```python
from build123d import *

# Parameters (mm, degrees)
CROQUIS1_W              = 10
CROQUIS1_H              = 8.5
SALIENTE_EXTRUIR1_DEPTH = 9.4
CROQUIS2_W              = 10
CROQUIS2_H              = 7
CORTAR_EXTRUIR1_DEPTH   = 6.2
CROQUIS3_W              = 0.25
CROQUIS3_H              = 8
CORTAR_EXTRUIR2_DEPTH   = 10
CROQUIS4_W              = 3
CROQUIS4_H              = 0.5
CORTAR_EXTRUIR3_DEPTH   = 10
CROQUIS5_W              = 4
CROQUIS5_H              = 1
CORTAR_EXTRUIR4_DEPTH   = 10
CROQUIS6_R              = 0.57
SALIENTE_EXTRUIR2_DEPTH = 7.3
REDONDEO2_R             = 0.5
CROQUIS7_W              = 1
CROQUIS7_H              = 1.5
CORTAR_EXTRUIR5_DEPTH   = 14.8
CROQUIS8_W              = 3
CROQUIS8_H              = 3.2
CORTAR_EXTRUIR6_DEPTH   = 1.5
CORTAR_EXTRUIR7_DEPTH   = 10


with BuildPart() as part:
    # Croquis1 → Saliente-Extruir1 (new body)
    with BuildSketch(Plane(origin=(0, 0, 0), x_dir=(1, 0, 0), z_dir=(0, 1, 0))):
        Rectangle(CROQUIS1_W, CROQUIS1_H)
    extrude(amount=SALIENTE_EXTRUIR1_DEPTH)

    # Croquis2 → Cortar-Extruir1 (cut)
    with BuildSketch(Plane(origin=(0, 9.4, 0), x_dir=(1, 0, 0), z_dir=(0, 1, 0))):
        with Locations((0, 0.75)):
            Rectangle(CROQUIS2_W, CROQUIS2_H)
    extrude(amount=-CORTAR_EXTRUIR1_DEPTH, mode=Mode.SUBTRACT)

    # Croquis3 → Cortar-Extruir2 (cut)
    with BuildSketch(Plane.ZY.offset(5)):
        with Locations((4.125, 4)):
            Rectangle(CROQUIS3_W, CROQUIS3_H)
    extrude(amount=-CORTAR_EXTRUIR2_DEPTH, mode=Mode.SUBTRACT)

    # Croquis4 → Cortar-Extruir3 (cut)
    with BuildSketch(Plane(origin=(0, 0, -4.25), x_dir=(-1, 0, 0), z_dir=(0, 0, -1))):
        with Locations((0, 0.25)):
            Rectangle(CROQUIS4_W, CROQUIS4_H)
    extrude(amount=-CORTAR_EXTRUIR3_DEPTH, mode=Mode.SUBTRACT)

    # Croquis5 → Cortar-Extruir4 (cut)
    with BuildSketch(Plane.ZY.offset(5)):
        with Locations((0.75, 0.5)):
            Rectangle(CROQUIS5_W, CROQUIS5_H)
    extrude(amount=-CORTAR_EXTRUIR4_DEPTH, mode=Mode.SUBTRACT)

    # Croquis6 → Saliente-Extruir2 (add, symmetric)
    with BuildSketch(Plane(origin=(0, 3.6, 0), x_dir=(1, 0, 0), z_dir=(0, 1, 0))):
        with Locations(Location((-2.5, -0.5, 0), (0, 0, 270))):
            Circle(CROQUIS6_R)
        with Locations(Location((2.5, -0.5, 0), (0, 0, 270))):
            Circle(CROQUIS6_R)
    extrude(amount=SALIENTE_EXTRUIR2_DEPTH, both=True)

    # Redondeo2
    redondeo2_edges = [part.edges().sort_by_distance(p)[0] for p in [
        (2.5, -3.7, -0.07),
        (2.5, 10.9, -0.07),
        (-2.5, -3.7, -0.07),
        (-2.5, 10.9, -0.07),
    ]]
    fillet(redondeo2_edges, radius=REDONDEO2_R)

    # Croquis7 → Cortar-Extruir5 (cut)
    with BuildSketch(Plane(origin=(0, 9.4, 0), x_dir=(1, 0, 0), z_dir=(0, 1, 0))):
        with Locations((-4.5, -3.5)):
            Rectangle(CROQUIS7_W, CROQUIS7_H)
        with Locations((4.5, -3.5)):
            Rectangle(CROQUIS7_W, CROQUIS7_H)
    extrude(amount=-CORTAR_EXTRUIR5_DEPTH, mode=Mode.SUBTRACT)

    # Croquis8 → Cortar-Extruir6 (cut)
    with BuildSketch(Plane.XY.offset(4)):
        with Locations((0, 1.6)):
            Rectangle(CROQUIS8_W, CROQUIS8_H)
    extrude(amount=-CORTAR_EXTRUIR6_DEPTH, mode=Mode.SUBTRACT)

    # Croquis9 → Cortar-Extruir7 (cut)
    with BuildSketch(Plane.ZY.offset(4)):
        Polygon((4.25, 8.6), (4.25, 9.4), (3.85, 9.4), align=None)
        Polygon((2.75, 8.5), (2.75, 9.4), (3.15, 9.4), align=None)
    extrude(amount=-CORTAR_EXTRUIR7_DEPTH, mode=Mode.SUBTRACT)


solid = part.part
```
Part model, mm, in its own coordinate system. A direction names the side the tool comes from. Round coordinates to 2 decimals unless told otherwise and drop trailing zeros. Loops run counter-clockwise (first coordinate to the right, second up) from the corner with the lowest first, then second, coordinate; pieces in that order, holes last. Notation, with made-up numbers: (49.25, 79.5) -> (95.25, 79.5) arc R20 cw to (95.25, 111.5) -> close; hole circle Ø6 at (-40, 45). An arc over 180 degrees is marked (long way). Use CSV: the item, a comma, the result in double quotes. Start each with the question number.
1) Cut at C-C, the plane x = -3.25. Write the cut outline in (y, z).
2) Drop flat-ended pins along their axis: P1, Ø1.1, axis at x = 4.5, y = 2.5, coming from the +Z side; P2, Ø1.4, axis at x = -2.5, z = 3.5, coming from the -Y side; P3, Ø3.5, axis at x = -1, z = -2, coming from the +Y side. Give the stop position or say it passes through.
3) Cut at B-B, the plane y = 6.5. Write the cut outline in (x, z).
4) Which spindle directions (+Z, -Z, +X, -X, +Y, -Y) get a long thin tool onto all of the face, cutting with end or side? Do faces 4 (the flat face through (-0.056, 8.956, 2.953)), 5 (the flat face through (3, 0, 3)), 6 (the flat face through (3, 0, -3)), 7 (the cylindrical face through (-2.85, -1.07, 0.05)). Say none if no direction does.
5) Cut at A-A, the plane x = -0.5. Write the cut outline in (y, z).
6) Wall check: L1, parallel to X at y = -0.5, z = 0.5; L2, parallel to Y at x = 2.25, z = -3.75; L3, parallel to X at y = 6.75, z = 3. Give the ranges that are in metal, low to high. Write a range as [from, to].
7) Cut at D-D, the plane y = 1.25. Write the cut outline in (x, z).
8) Pull direction Z, two halves, no side cores. Call faces 1 (the flat face through (5, 2, -1)), 2 (the flat face through (0, 4, 4)), 3 (the flat face through (-0.1, 0.7, -1.25)): +Z half, -Z half, draft (parallel to the pull), parting line (faces both ways), or undercut.
Determined:
1,outline,"(0, -4.25) -> (3.2, -4.25) -> (3.2, 2.75) -> (8.5, 2.75) -> (9.4, 3.15) -> (9.4, 3.85) -> (8.6, 4.25) -> (8, 4.25) -> (8, 4) -> (0, 4) -> (0, 2.75) -> (1, 2.75) -> (1, -1.25) -> (0, -1.25) -> close"
2,P1,"stops at z = 4"
2,P2,"stops at y = 0"
2,P3,"stops at y = 3.2"
3,outline,"(-4, 2.75) -> (4, 2.75) -> (4, 4) -> (-4, 4) -> close; circle Ø1.14 at (-2.5, 0.5); circle Ø1.14 at (2.5, 0.5)"
4,face 4,"+X, -X, +Y"
4,face 5,"+Z, +X, -X, -Y"
4,face 6,"-Z, +X, -X, -Y"
4,face 7,"-Y"
5,outline,"(0.5, -4.25) -> (3.2, -4.25) -> (3.2, 2.5) -> (1, 2.5) -> (1, -1.25) -> (0.5, -1.25) -> close; (3.2, 2.75) -> (8.5, 2.75) -> (9.4, 3.15) -> (9.4, 3.85) -> (8.6, 4.25) -> (8, 4.25) -> (8, 4) -> (3.2, 4) -> close"
6,L1,"x = [-3.07, -1.93], [1.93, 3.07]"
6,L2,"y = [0, 3.2]"
6,L3,"x = [-4, 4]"
7,outline,"(-5, -4.25) -> (5, -4.25) -> (5, 2.75) -> (4, 2.75) -> (4, 4) -> (1.5, 4) -> (1.5, 2.5) -> (-1.5, 2.5) -> (-1.5, 4) -> (-4, 4) -> (-4, 2.75) -> (-5, 2.75) -> close"
8,face 1,"draft"
8,face 2,"+Z half"
8,face 3,"undercut"
